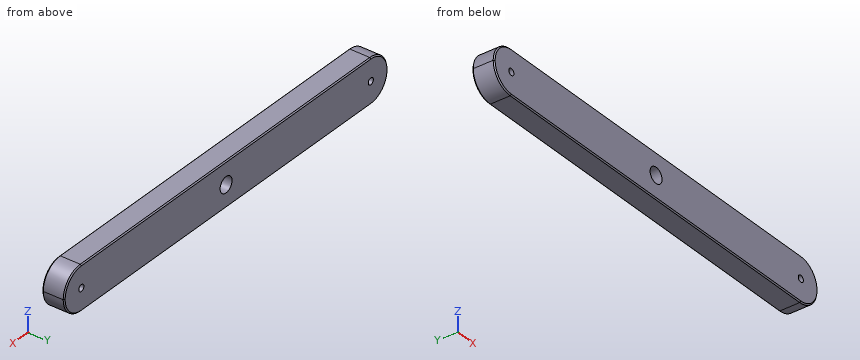
Autodesk Inventor part; units mm, degrees
ref_plane "YZ Plane" through (0, 0, 0) normal (1, 0, 0) x (0, 1, 0)
ref_plane "XZ Plane" through (0, 0, 0) normal (0, 1, 0) x (-1, 0, 0)
ref_plane "XY Plane" through (0, 0, 0) normal (0, 0, 1) x (1, 0, 0)
sketch "Sketch1" plane through (0, 0, 0) normal (0, 1, 0) x (-1, 0, 0)
  line L0 (-95, 10) -> (95, 10)
  line L1 (95, 10) -> (95, -10)
  line L2 (95, -10) -> (-95, -10)
  line L3 (-95, -10) -> (-95, 10)
  line L4 (-95, 10) -> (95, -10) construction
  line L5 (95, 10) -> (-95, -10) construction
  point P0 (0, 0)
  dimension "Length" = 190
  dimension "Width" = 20
extrude "Extrusion1" add sketch "Sketch1" along normal mid plane 10
sketch "Sketch2" plane through (0, 5, 0) normal (0, 1, 0) x (1, 0, 0)
  circle A0 centre (0, 0) radius 3.5
  dimension "d4" = 7
extrude "Extrusion2" cut sketch "Sketch2" against normal up to surface (10 mm away)
sketch "Sketch3" plane through (0, 5, 0) normal (0, 1, 0) x (1, 0, 0)
  circle A0 centre (0, 0) radius 3.5
  point P0 (-15, 0)
  point P1 (15, 0)
  dimension "d7" = 30
  dimension "d8" = 15
hole "Hole1" [suppressed]
sketch "Sketch4" plane through (0, 5, 0) normal (0, 1, 0) x (1, 0, 0)
  point P0 (0, 0)
  point P1 (-85, 0)
  point P2 (85, 0)
  dimension "d16" = 170
  dimension "d17" = 85
hole "Hole2" at (-85, 5, 0) at (85, 5, 0) direction (0, -1, 0) diameter 3 end through all
fillet "Fillet1" radius 10 4 edges at (95, 0, 10) (95, 0, -10) (-95, 0, 10) (-95, 0, -10)
chamfer "Chamfer1" distance 0.5 angle 45 8 edges at (0, 5, 10) (92.0712, 5, 7.0712) (0, 5, -10) (-92.0712, 5, 7.0712) (0, -5, 10) (-92.0712, -5, 7.0712) (0, -5, -10) (92.0712, -5, 7.0712)
properties part number "Lower Arm Brass Plate - 2" material "Brass, Soft Yellow"
Here's how the part is built. I have some questions about the finished solid (model axes, mm). Give positions to 0.01 mm unless a question says otherwise; leave off trailing zeros. Loops run counter-clockwise (first coordinate to the right, second up) from the corner with the lowest first, then second, coordinate; pieces in that order, holes last. Notation, with made-up numbers: (38, 15.5) -> (58, 15.5) arc R14 ccw to (58, 35.5) -> close; hole circle Ø2 at (33.5, -3.75). An arc over 180 degrees is marked (long way). One line per item, written item: value.
Q1. Suppose I cut it at A-A on x = 0. Please give me the cut outline in (y, z), then the cut area to 4 significant figures.
Answers follow:
outline: (-5, -9.5) -> (-4.5, -10) -> (4.5, -10) -> (5, -9.5) -> (5, -3.5) -> (-5, -3.5) -> close; (-5, 3.5) -> (5, 3.5) -> (5, 9.5) -> (4.5, 10) -> (-4.5, 10) -> (-5, 9.5) -> close
area: 129.5 mm^2
Q2. Suppose I cut it at B-B on y = -1.5. State how many separate pieces and enclosed holes the cut face has, then the cut area to 3 significant figures.
Answers follow:
separate pieces: 1
enclosed holes: 3
area: 3,660 mm^2
Q3. If I drill on line 1 along X through (y, z) = (-1, 0); line 2 along Z through (x, y) = (-85, 0.5); line 3 along Z through (x, y) = (0, 2.75), over which ranges is the centre line in solid material (lowest first)?
Answers follow:
line 1: -95 to -86.5, -83.5 to -3.5, 3.5 to 83.5, 86.5 to 95
line 2: -10 to -1.5, 1.5 to 10
line 3: -10 to -3.5, 3.5 to 10
Q4. I'm going to push flat-ended pins straight in: pin 1 Ø5.5 at (x, z) = (0, 0) entering from +Y; pin 2 Ø2 at (y, z) = (-2, 4) entering from -X; pin 3 Ø2 at (y, z) = (3.5, -1.5) entering from +X. Where does each tip first touch, or does it pass through?
Answers follow:
pin 1: through
pin 2: x = -94.54
pin 3: x = 94.99
